Read the model definition and answer for the solid it produces. Units are mm, in the model's axes. A direction names the side the tool comes from. Coordinates: 2 decimals unless noted, no trailing zeros. Write each loop counter-clockwise with the first axis right and the second up, starting at its lowest first coordinate (ties: lowest second). Pieces come first, ordered by that corner, then holes.
1) The part is cut by section A-A (y = 37). Determine the outline of the cut face in (x, z).
2) The part is cut by section C-C (x = 4.5). Determine the outline of the cut face in (y, z), then the cut area to 3 significant figures.
3) Find the intervals of material crossed by line 1 (X direction, y = 20, z = 21.5), in increasing order.
4) Which of the six approach directions +Z, -Z, +X, -X, +Y, -Y give full straight-line access (tool end or side, diameter ignored) to faces 1 (the face through (0.7, 25.9, 307.3)), 2 (the face through (1.5, 16, 172)), 3 (the face through (14, 1, 349.2))?
5) The part is cut by section B-B (z = 109.5). Determine the outline of the cut face in (x, y), then the cut area to 3 significant figures.
6) Each of these flat-tipped pins is pushed along its axis until it touches: pin 1 Ø10 at (x, z) = (20, 158) entering from +Y; pin 2 Ø0.8 at (x, z) = (1, 229.5) entering from +Y; pin 3 Ø15 at (y, z) = (18.5, 135) entering from +X. Where does it stop, or does it pass through?
from build123d import *

# Parameters (mm, degrees)
SALIENTE_EXTRUIR1_DEPTH    = 349.2
CROQUIS5_W                 = 275.2
CROQUIS5_H                 = 30
CORTAR_EXTRUIR2_DEPTH      = 1
CORTAR_EXTRUIR2_DEPTH_BACK = 2
CHAFL_N1_SIZE              = 10


with BuildPart() as part:
    # Croquis1 → Saliente-Extruir1 (new body)
    with BuildSketch(Plane.XY):
        Polygon((0, 0), (0, 50.8), (1.5, 50.8), (1.5, 1.5), (50.8, 1.5), (50.8, 0), align=None)
    extrude(amount=SALIENTE_EXTRUIR1_DEPTH)

    # Croquis5 → Cortar-Extruir2 (cut, two sides)
    with BuildSketch(Plane.ZY) as cortar_extruir2_sk:
        with Locations((174.6, 35.8)):
            Rectangle(CROQUIS5_W, CROQUIS5_H)
    extrude(amount=CORTAR_EXTRUIR2_DEPTH, mode=Mode.SUBTRACT)
    extrude(cortar_extruir2_sk.sketch, amount=-CORTAR_EXTRUIR2_DEPTH_BACK, mode=Mode.SUBTRACT)

    # Chaflán1
    chafl_n1_edges = [part.edges().sort_by_distance(p)[0] for p in [
        (0.75, 20.8, 37),
        (0.75, 20.8, 312.2),
        (0.75, 50.8, 312.2),
        (0.75, 50.8, 37),
    ]]
    chamfer(chafl_n1_edges, length=CHAFL_N1_SIZE)


solid = part.part
Reported:
1. outline: (0, 0) - (1.5, 0) - (1.5, 37) - (0, 37) - close; (0, 312.2) - (1.5, 312.2) - (1.5, 349.2) - (0, 349.2) - close
2. outline: (0, 0) - (1.5, 0) - (1.5, 349.2) - (0, 349.2) - close
2. area: 524 mm2
3. line 1: x = 0 to 1.5
4. face 1: +X, -X, +Y
4. face 2: +Z, -Z, +X, +Y
4. face 3: +Z, +X, -X, +Y, -Y
5. outline: (0, 0) - (50.8, 0) - (50.8, 1.5) - (1.5, 1.5) - (1.5, 20.8) - (0, 20.8) - close
5. area: 105 mm2
6. pin 1: stops at y = 1.5
6. pin 2: stops at y = 20.8
6. pin 3: stops at x = 1.5
